```python
from build123d import *

# Parameters (mm, degrees)
F1_DEPTH  = 10
F2_R      = 4
F3_DEPTH  = 38
F4_R      = 4
F5_DEPTH  = 70
F8_DEPTH  = 10
F9_R      = 4
F10_DEPTH = 40
F11_R     = 4
F12_DEPTH = 100
F13_DEPTH = 5
F14_R     = 2
F15_DEPTH = 10
F16_SIZE  = 2


with BuildPart() as f1:
    # F0 (on Front) → F1 (new body)
    with BuildSketch(Plane.XZ):
        Polygon((19, 24), (-19, 24), (-19, 9), (-35, 9), (-35, -24), (35, -24), (35, 9), (19, 9), align=None)
    extrude(amount=F1_DEPTH)

    # F2 (on face) → F3 (cut)
    with BuildSketch(Plane.YZ.offset(19)):
        with Locations((-5, 19)):
            Circle(F2_R)
    extrude(amount=-F3_DEPTH, mode=Mode.SUBTRACT)

    # F4 (on face) → F5 (cut)
    with BuildSketch(Plane.YZ.offset(35)):
        with Locations((-5, -19)):
            Circle(F4_R)
    extrude(amount=-F5_DEPTH, mode=Mode.SUBTRACT)


with BuildPart() as f8:
    # F7 (on Front) → F8 (new body)
    with BuildSketch(Plane.XZ):
        Polygon((18, 24), (-18, 24), (-18, 9), (-39, 9), (-39, -24), (39, -24), (39, 9), (18, 9), align=None)
    extrude(amount=F8_DEPTH)

    # F9 (on face) → F10 (cut)
    with BuildSketch(Plane.YZ.offset(18)):
        with Locations((-5, 19)):
            Circle(F9_R)
    extrude(amount=-F10_DEPTH, mode=Mode.SUBTRACT)

    # F11 (on face) → F12 (cut)
    with BuildSketch(Plane.YZ.offset(39)):
        with Locations((-5, -19)):
            Circle(F11_R)
    extrude(amount=-F12_DEPTH, mode=Mode.SUBTRACT)

    # F13 (add): a face of the model
    f13_faces = [f8.faces().sort_by_distance(p)[0] for p in [
        (0, -5, 24),
    ]]
    extrude(f13_faces, amount=F13_DEPTH)

    # F14 (on face) → F15 (cut)
    with BuildSketch(Plane.XY.offset(29)):
        with Locations((0, -5)):
            Circle(F14_R)
    extrude(amount=-F15_DEPTH, mode=Mode.SUBTRACT)

    # F16
    f16_edges = [f8.edges().sort_by_distance(p)[0] for p in [
        (0, -10, 29),
        (0, 0, 29),
    ]]
    chamfer(f16_edges, length=F16_SIZE)


solid = f8.part
```
The model under review builds one solid part; all positions refer to its coordinate system, in mm. A direction names the side the tool comes from. Round coordinates to 2 decimals unless told otherwise and drop trailing zeros. Loops run counter-clockwise (first coordinate to the right, second up) from the corner with the lowest first, then second, coordinate; pieces in that order, holes last.
1) Consider section B-B on x = 0. State the section outline as (y, z) points, then the cut area to 3 significant figures.
Values follow:
outline: (-10, -24) - (0, -24) - (0, 27) - (-2, 29) - (-3, 29) - (-3, 22.46) arc R4 cw (long way) to (-7, 22.46) - (-7, 29) - (-8, 29) - (-10, 27) - close; hole circle Ø8 at (-5, -19)
area: 401 mm2
2) Consider section A-A on z = 19. State the section outline as (x, y) points.
Values follow:
outline: (-18, -10) - (18, -10) - (18, -9) - (-18, -9) - close; (-18, -1) - (18, -1) - (18, 0) - (-18, 0) - close
3) The part is to be moulded in two halves that separate along Z. For faces 1 (the face through (18, -1.6, 16.6)), 2 (the face through (0, -9, 28)), 3 (the face through (0.252, -5.867, 15.095)), say which applies: pulls with the +Z half, pulls with the -Z half, needs draft (parallel to the pull), parting line crosses it, or undercut.
Values follow:
face 1: needs draft
face 2: pulls with the +Z half
face 3: undercut
4) Consider section D-D on x = -16. State the section outline as (y, z) points, then the cut area to 3 significant figures.
Values follow:
outline: (-10, -24) - (0, -24) - (0, 27) - (-2, 29) - (-8, 29) - (-10, 27) - close; hole circle Ø8 at (-5, -19); hole circle Ø8 at (-5, 19)
area: 425 mm2
5) Consider section C-C on y = -5. State the section outline as (x, z) points.
Values follow:
outline: (-39, -24) - (39, -24) - (39, -23) - (-39, -23) - close; (-39, -15) - (39, -15) - (39, 9) - (18, 9) - (18, 15) - (-18, 15) - (-18, 9) - (-39, 9) - close; (-18, 23) - (-2, 23) - (-2, 29) - (-18, 29) - close; (2, 23) - (18, 23) - (18, 29) - (2, 29) - close
6) Clearance check with flat-ended pins moving along their axes: P1, Ø5, axis at y = -5.5, z = 21.5, coming from the -X side; P2, Ø5, axis at y = -3, z = 21.5, coming from the +X side; P3, Ø1.5, axis at x = -25.5, y = -5, coming from the +Z side. State where each tip first meets the part, or that it passes through.
Values follow:
P1: stops at x = -18
P2: stops at x = 18
P3: stops at z = 9
7) Tool access review of faces 4 (the face through (29, -5, 9)), 5 (the face through (-2, -5, 26)), 6 (the face through (-18, -1.6, 16.6)): name each direction out of +Z, -Z, +X, -X, +Y, -Y from which nothing blocks a thin tool from reaching the whole face with its end or side.
Values follow:
face 4: +Z, +X, +Y, -Y
face 5: +Z
face 6: +Z, -X, +Y, -Y
8) Wall thickness on line 1 along Z through (x, y) = (-8, -4.75); line 2 along Z through (x, y) = (8.5, -6.5); line 3 along X through (y, z) = (-5, 26.75): over which ranges is each line inside the solid? List them lowest first.
Values follow:
line 1: z = -24 to -22.99, -15.01 to 15.01, 22.99 to 29
line 2: z = -24 to -22.71, -15.29 to 15.29, 22.71 to 29
line 3: x = -18 to -2, 2 to 18
